Check sheet for the drawn part. Datum: minimum x, y, z corner. Units: mm. Give positions to 0.01 mm unless a question says otherwise; leave off trailing zeros. Loops run counter-clockwise (first coordinate to the right, second up) from the corner with the lowest first, then second, coordinate; pieces in that order, holes last. Notation, with made-up numbers: (82.25, 43) - (101.25, 43) arc R31 ccw to (101.25, 79) - close; hole circle Ø10 at (80, -0.5). An arc over 180 degrees is marked (long way). Use one line per item in the form item = value.
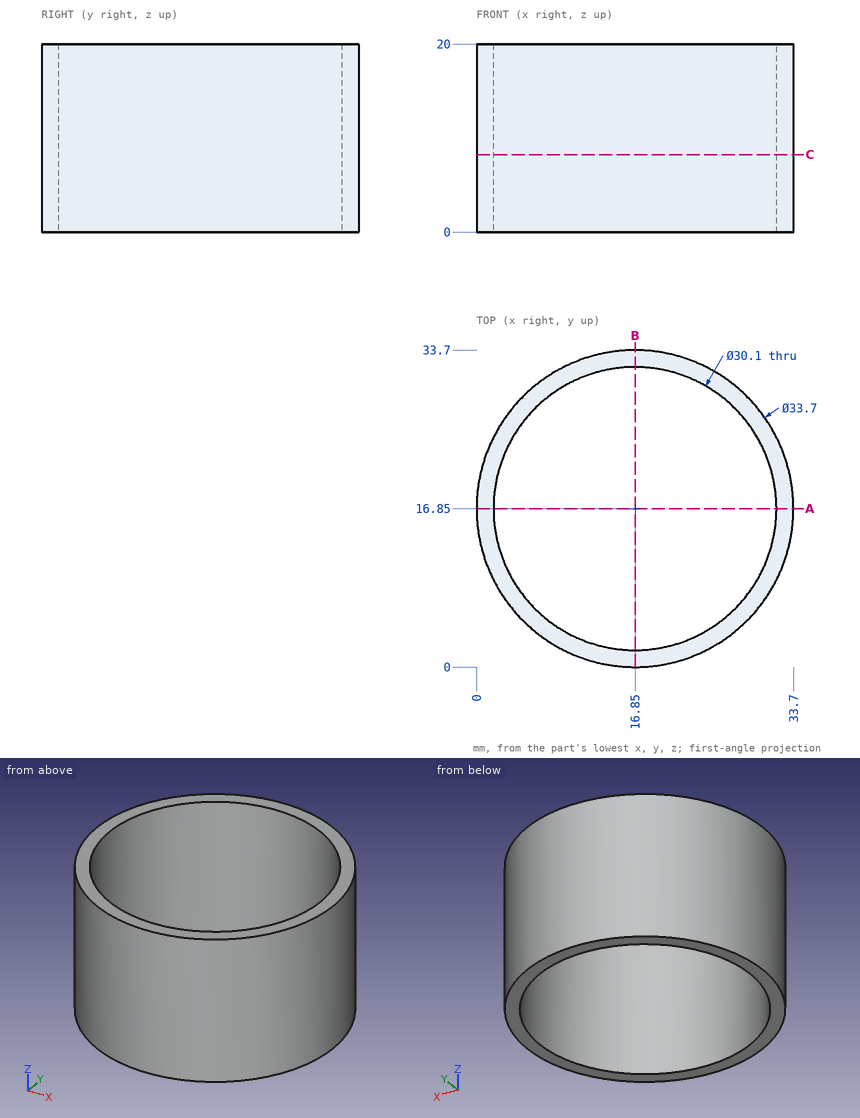
1. Section check A-A, the plane y = 16.85. Record the cut outline in (x, z).
Result set:
outline = (0, 0) - (1.8, 0) - (1.8, 20) - (0, 20) - close; (31.9, 0) - (33.7, 0) - (33.7, 20) - (31.9, 20) - close
2. Scan lines: probe 1 along Y at (x, z) = (16.85, 14.5); probe 2 along X at (y, z) = (30, 6.75); probe 3 along X at (y, z) = (10, 14.5). Record each from-to range of solid material in increasing order.
Result set:
probe_1 = 0 to 1.8, 31.9 to 33.7
probe_2 = 6.31 to 9.53, 24.17 to 27.39
probe_3 = 1.46 to 3.45, 30.25 to 32.24
3. Section check C-C, the plane z = 8.25. Record the cut outline in (x, y), then the cut area to 3 significant figures.
Result set:
outline = circle Ø33.7 at (16.85, 16.85); hole circle Ø30.1 at (16.85, 16.85)
area = 180 mm²
4. Depth check by flat-ended pin: pin 1 Ø10 at (x, z) = (27, 17.5) entering from -Y; pin 2 Ø6 at (y, z) = (4.5, 17.5) entering from -X; pin 3 Ø1.5 at (y, z) = (9, 6) entering from -X. Enter the tip coordinate at first touch or a pass-through.
Result set:
pin_1 = 0.81
pin_2 = 2.83
pin_3 = 1.57
